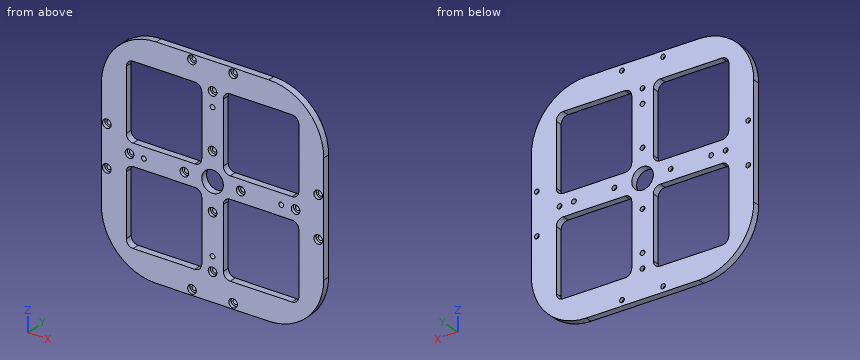
```python
from build123d import *

# Parameters (mm, degrees)
SKETCH1_W                = 205.74
SKETCH1_H                = 205.74
SKETCH1_R                = 2.200000045
BOSS_EXTRUDE1_DEPTH      = 6.35
SKETCH3_R                = 9.999999939
CUT_EXTRUDE2_DEPTH       = 146.618667416
SKETCH4_W                = 69.85
SKETCH4_H                = 69.85
CUT_EXTRUDE3_DEPTH       = 146.618667416
FILLET1_R                = 6.35
CIRPATTERN2_COUNT        = 4
FILLET1_OF_CIRPATTERN2_R = 6.35
FILLET2_R                = 50.8
SKETCH10_R               = 2.200000045
CUT_EXTRUDE6_DEPTH       = 146.618667416
SKETCH11_R               = 4.000000001
CUT_EXTRUDE7_DEPTH       = 3.000000096
CIRPATTERN4_COUNT        = 4


with BuildPart() as part:
    # Sketch1 → Boss-Extrude1 (new body)
    with BuildSketch(Plane(origin=(0, 0, 0), x_dir=(1, 0, 0), z_dir=(0, 1, 0))):
        Rectangle(SKETCH1_W, SKETCH1_H)
        with Locations(Location((63.5, 0, 0), (0, 0, 270))):
            Circle(SKETCH1_R, mode=Mode.SUBTRACT)
        with Locations(Location((0, -63.5, 0), (0, 0, 270))):
            Circle(SKETCH1_R, mode=Mode.SUBTRACT)
        with Locations(Location((-63.5, 0, 0), (0, 0, 270))):
            Circle(SKETCH1_R, mode=Mode.SUBTRACT)
        with Locations(Location((0, 63.5, 0), (0, 0, 270))):
            Circle(SKETCH1_R, mode=Mode.SUBTRACT)
    extrude(amount=BOSS_EXTRUDE1_DEPTH)

    # Sketch3 → Cut-Extrude2 (cut, through all)
    with BuildSketch(Plane(origin=(0, 6.35, 0), x_dir=(1, 0, 0), z_dir=(0, 1, 0))):
        with Locations(Location((0, 0, 0), (0, 0, 270))):
            Circle(SKETCH3_R)
    extrude(amount=-CUT_EXTRUDE2_DEPTH, mode=Mode.SUBTRACT)

    # Sketch4 → Cut-Extrude3 (cut, through all)
    with BuildSketch(Plane(origin=(0, 6.35, 0), x_dir=(1, 0, 0), z_dir=(0, 1, 0))):
        with Locations((-44.901280605, 44.901280605)):
            Rectangle(SKETCH4_W, SKETCH4_H)
    cut_extrude3 = extrude(amount=-CUT_EXTRUDE3_DEPTH, mode=Mode.SUBTRACT)

    # Fillet1
    fillet1_edges = [part.edges().sort_by_distance(p)[0] for p in [
        (-9.976280605, 3.175, -79.826280605),
        (-9.976280605, 3.175, -9.976280605),
        (-79.826280605, 3.175, -9.976280605),
        (-79.826280605, 3.175, -79.826280605),
    ]]
    fillet(fillet1_edges, radius=FILLET1_R)

    # CirPattern2: Cut-Extrude3 ×4 about axis
    cirpattern2_axis = Axis((0, 0, 0), (0, 1, 0))
    for i in range(1, CIRPATTERN2_COUNT):
        add(cut_extrude3.rotate(cirpattern2_axis, i * 360 / CIRPATTERN2_COUNT), mode=Mode.SUBTRACT)

    # Fillet1 of CirPattern2
    fillet1_of_cirpattern2_edges = [part.edges().sort_by_distance(p)[0] for p in [
        (-79.826280605, 3.175, 9.976280605),
        (-9.976280605, 3.175, 9.976280605),
        (-9.976280605, 3.175, 79.826280605),
        (-79.826280605, 3.175, 79.826280605),
        (9.976280605, 3.175, 79.826280605),
        (9.976280605, 3.175, 9.976280605),
        (79.826280605, 3.175, 9.976280605),
        (79.826280605, 3.175, 79.826280605),
        (79.826280605, 3.175, -9.976280605),
        (9.976280605, 3.175, -9.976280605),
        (9.976280605, 3.175, -79.826280605),
        (79.826280605, 3.175, -79.826280605),
    ]]
    fillet(fillet1_of_cirpattern2_edges, radius=FILLET1_OF_CIRPATTERN2_R)

    # Fillet2
    fillet2_edges = [part.edges().sort_by_distance(p)[0] for p in [
        (102.87, 3.175, 102.87),
        (-102.87, 3.175, 102.87),
        (-102.87, 3.175, -102.87),
        (102.87, 3.175, -102.87),
    ]]
    fillet(fillet2_edges, radius=FILLET2_R)

    # Sketch10 → Cut-Extrude6 (cut, through all)
    with BuildSketch(Plane(origin=(0, 6.35, 0), x_dir=(1, 0, 0), z_dir=(0, 1, 0))):
        with Locations(Location((0, -26.035, 0), (0, 0, 270))):
            Circle(SKETCH10_R)
        with Locations(Location((0, -76.835, 0), (0, 0, 270))):
            Circle(SKETCH10_R)
        with Locations(Location((-19.05, -97.79, 0), (0, 0, 270))):
            Circle(SKETCH10_R)
        with Locations(Location((19.05, -97.79, 0), (0, 0, 270))):
            Circle(SKETCH10_R)
    cut_extrude6 = extrude(amount=-CUT_EXTRUDE6_DEPTH, mode=Mode.SUBTRACT)

    # Sketch11 → Cut-Extrude7 (cut)
    with BuildSketch(Plane.XZ):
        with Locations(Location((-19.05, 97.79, 0), (0, 0, 270))):
            Circle(SKETCH11_R)
        with Locations(Location((19.05, 97.79, 0), (0, 0, 270))):
            Circle(SKETCH11_R)
        with Locations(Location((0, 76.835, 0), (0, 0, 270))):
            Circle(SKETCH11_R)
        with Locations(Location((0, 26.035, 0), (0, 0, 270))):
            Circle(SKETCH11_R)
    cut_extrude7 = extrude(amount=-CUT_EXTRUDE7_DEPTH, mode=Mode.SUBTRACT)

    # CirPattern4: Cut-Extrude6, Cut-Extrude7 ×4 about axis
    cirpattern4_axis = Axis((0, 0, 0), (0, 1, 0))
    add([cut_extrude6.rotate(cirpattern4_axis, i * 360 / CIRPATTERN4_COUNT) for i in range(1, CIRPATTERN4_COUNT)], mode=Mode.SUBTRACT)
    add([cut_extrude7.rotate(cirpattern4_axis, i * 360 / CIRPATTERN4_COUNT) for i in range(1, CIRPATTERN4_COUNT)], mode=Mode.SUBTRACT)


solid = part.part
```
The listing builds one solid part. Answer for the finished solid, in the listing's coordinates (mm). Round coordinates to 2 decimals unless told otherwise and drop trailing zeros. Order: outer loops, then holes, each group sorted by start corner. A loop starts at its lowest first (then second) coordinate and runs counter-clockwise, first axis right, second up. Notation, with made-up numbers: (-12.5, 44) -> (-6.5, 44) arc R36 cw to (-6.5, 80) -> close; hole circle Ø5 at (20.5, 47). An arc over 180 degrees is marked (long way). Answer as CSV lines item,"result". Start each with the question number.
(1) The part is cut by section A-A (x = -37.5). Determine the outline of the cut face in (y, z).
(2) The part is cut by section C-C (y = 5.25). Count the separate pieces of the cut face and the enclosed holes in it, then the cut area to 3 significant figures.
(3) Flat-ended cylindrical pins translate along their axes: pin 1 Ø3 at (x, y) = (-76, 4) entering from +Z; pin 2 Ø3.5 at (x, z) = (-19.05, -97.79) entering from +Y; pin 3 Ø5.5 at (x, z) = (97.79, 19.05) entering from -Y. Find the tip coordinate at first contact, or state that the pin passes through.
(4) The part is cut by section B-B (z = 49.5). Determine the outline of the cut face in (x, y).
(5) Find the intervals of material crossed by probe 1 along X at (y, z) = (4.5, -21.5); probe 2 along X at (y, z) = (1.5, -67), in increasing order. Write a range as from..to.
Evaluation:
1,outline,"(0, -102.87) -> (6.35, -102.87) -> (6.35, -79.83) -> (0, -79.83) -> close; (0, -9.98) -> (6.35, -9.98) -> (6.35, 9.98) -> (0, 9.98) -> close; (0, 79.83) -> (6.35, 79.83) -> (6.35, 102.87) -> (0, 102.87) -> close"
2,separate pieces,"1"
2,enclosed holes,"25"
2,area,"20,100 mm²"
3,pin 1,"z = 97.65"
3,pin 2,"through"
3,pin 3,"y = 3"
4,outline,"(-102.87, 0) -> (-79.83, 0) -> (-79.83, 6.35) -> (-102.87, 6.35) -> close; (-9.98, 0) -> (9.98, 0) -> (9.98, 6.35) -> (-9.98, 6.35) -> close; (79.83, 0) -> (102.87, 0) -> (102.87, 6.35) -> (79.83, 6.35) -> close"
5,probe 1,"-102.87..-79.83, -9.98..9.98, 79.83..102.87"
5,probe 2,"-100.63..-79.83, -9.98..9.98, 79.83..100.63"
